Could you check a few things on this model? Use its own coordinates, in mm. A direction names the side the tool comes from. Round coordinates to 2 decimals unless told otherwise and drop trailing zeros. Order: outer loops, then holes, each group sorted by start corner. A loop starts at its lowest first (then second) coordinate and runs counter-clockwise, first axis right, second up. Notation, with made-up numbers: (79, 36.25) - (94, 36.25) arc R4 cw to (94, 43.25) - close; hole circle Ø6 at (65, 12.5). An arc over 180 degrees is marked (long way). Use one line per item in the form item = value.
from build123d import *

# Parameters (mm, degrees)
BOSS_EXTRUDE1_DEPTH = 50.8


with BuildPart() as part:
    # Sketch1 → Boss-Extrude1 (new body)
    with BuildSketch(Plane(origin=(0, 0, 0), x_dir=(1, 0, 0), z_dir=(0, 1, 0))):
        with BuildLine():
            Line((-1.27, 3.175), (-1.27, 38.735))
            Line((-1.27, 38.735), (1.27, 38.735))
            Line((1.27, 38.735), (1.27, 3.175))
            ThreePointArc((1.27, 3.175), (1.709789826, 2.961442849), (2.114630657, 2.687352263))
            Line((2.114630657, 2.687352263), (32.910494016, 20.467352263))
            Line((32.910494016, 20.467352263), (34.180494016, 18.267647737))
            Line((34.180494016, 18.267647737), (3.384630657, 0.487647737))
            ThreePointArc((3.384630657, 0.487647737), (3.419579653, 0), (3.384630657, -0.487647737))
            Line((3.384630657, -0.487647737), (34.180494016, -18.267647737))
            Line((34.180494016, -18.267647737), (32.910494016, -20.467352263))
            Line((32.910494016, -20.467352263), (2.114630657, -2.687352263))
            ThreePointArc((2.114630657, -2.687352263), (1.709789826, -2.961442849), (1.27, -3.175))
            Line((1.27, -3.175), (1.27, -38.735))
            Line((1.27, -38.735), (-1.27, -38.735))
            Line((-1.27, -38.735), (-1.27, -3.175))
            ThreePointArc((-1.27, -3.175), (-1.709789826, -2.961442849), (-2.114630657, -2.687352263))
            Line((-2.114630657, -2.687352263), (-32.910494016, -20.467352263))
            Line((-32.910494016, -20.467352263), (-34.180494016, -18.267647737))
            Line((-34.180494016, -18.267647737), (-3.384630657, -0.487647737))
            ThreePointArc((-3.384630657, -0.487647737), (-3.419579653, 0), (-3.384630657, 0.487647737))
            Line((-3.384630657, 0.487647737), (-34.180494016, 18.267647737))
            Line((-34.180494016, 18.267647737), (-32.910494016, 20.467352263))
            Line((-32.910494016, 20.467352263), (-2.114630657, 2.687352263))
            ThreePointArc((-2.114630657, 2.687352263), (-1.709789826, 2.961442849), (-1.27, 3.175))
        make_face()
    extrude(amount=BOSS_EXTRUDE1_DEPTH)


solid = part.part
Item 1: Imagine slicing it at B-B on z = 10. Please give me the cut outline in (x, y).
Found:
outline = (-19.86, 0) - (-14.78, 0) - (-14.78, 50.8) - (-19.86, 50.8) - close; (-1.27, 0) - (1.27, 0) - (1.27, 50.8) - (-1.27, 50.8) - close; (14.78, 0) - (19.86, 0) - (19.86, 50.8) - (14.78, 50.8) - close
Item 2: Imagine slicing it at A-A on y = 16. Please give me the cut outline in (x, z) (1 decimal), plus the area to 3 significant figures.
Found:
outline = (-34.2, -18.3) - (-32.9, -20.5) - (-2.1, -2.7) arc R3.4 ccw to (-1.3, -3.2) - (-1.3, -38.7) - (1.3, -38.7) - (1.3, -3.2) arc R3.4 ccw to (2.1, -2.7) - (32.9, -20.5) - (34.2, -18.3) - (3.4, -0.5) arc R3.4 ccw to (3.4, 0.5) - (34.2, 18.3) - (32.9, 20.5) - (2.1, 2.7) arc R3.4 ccw to (1.3, 3.2) - (1.3, 38.7) - (-1.3, 38.7) - (-1.3, 3.2) arc R3.4 ccw to (-2.1, 2.7) - (-32.9, 20.5) - (-34.2, 18.3) - (-3.4, 0.5) arc R3.4 ccw to (-3.4, -0.5) - close
area = 576 mm2
Item 3: I need wall thicknesses on L1, parallel to X at y = 4, z = 19.5 (3 decimals); L2, parallel to X at y = 17, z = 16; L3, parallel to Z at x = -15, y = 21. Which ranges of each line are inside material? Lowest first, please.
Found:
L1 = -33.469 to -31.235, -1.27 to 1.27, 31.235 to 33.469
L2 = -30.25 to -25.17, -1.27 to 1.27, 25.17 to 30.25
L3 = -10.13 to -7.19, 7.19 to 10.13
Item 4: Imagine slicing it at D-D on z = 28. Please give me the cut outline in (x, y), plus the area to 3 significant figures.
Found:
outline = (-1.27, 0) - (1.27, 0) - (1.27, 50.8) - (-1.27, 50.8) - close
area = 129 mm2
Item 5: Imagine slicing it at C-C on x = 14. Please give me the cut outline in (y, z).
Found:
outline = (0, -9.55) - (50.8, -9.55) - (50.8, -6.62) - (0, -6.62) - close; (0, 6.62) - (50.8, 6.62) - (50.8, 9.55) - (0, 9.55) - close
Item 6: For faces 1 (the face through (1.27, 25, 21)), 2 (the face through (18.567, 25.044, 9.253)), 3 (the face through (-17.728, 25.044, -11.702)), which set-ups out of +Z, -Z, +X, -X, +Y, -Y let a thin tool reach every point of the face, with its end or its side?
Found:
face_1 = +Z, +Y, -Y
face_2 = +X, +Y, -Y
face_3 = -Z, +Y, -Y
Item 7: Will these pins go through, and if not, where does the flat tip stop? P1, Ø8, axis at x = 26, y = 30.5, coming from the -Z side; P2, Ø4, axis at y = 12.5, z = 14, coming from the +X side; P3, Ø3, axis at x = -17.5, y = 34, coming from the -Z side; P4, Ø10, axis at x = -15.5, z = 18, coming from the +Y side.
Found:
P1 = -18.79
P2 = 30.25
P3 = -12.44
P4 = through
Item 8: If we mould it in two halves opening along X, with no side actions, what happens to faces 4 (the face through (18.998, 25.044, -9.502)), 5 (the face through (1.27, 25, -21)), 6 (the face through (-18.567, 25.044, -9.253))? For each: released by +X, released by -X, zero draft, split by the parting line, or undercut.
Found:
face_4 = released by +X
face_5 = undercut
face_6 = released by -X
